from build123d import *

# Parameters (mm, degrees)
SKETCH3_W           = 13
SKETCH3_H           = 120
BOSS_EXTRUDE1_DEPTH = 4
SKETCH11_W          = 33
SKETCH11_H          = 120
BOSS_EXTRUDE4_DEPTH = 4
SKETCH12_R          = 2.5
CUT_EXTRUDE3_DEPTH  = 76.305579191
SKETCH13_W          = 6.102814475
SKETCH13_H          = 45
CUT_EXTRUDE4_DEPTH  = 76.305579191


with BuildPart() as part:
    # Sketch3 → Boss-Extrude1 (new body)
    with BuildSketch(Plane.XY):
        with Locations((20.835766423, 0)):
            Rectangle(SKETCH3_W, SKETCH3_H)
        with BuildLine():
            Line((14.335766423, 0), (14.335766423, 60))
            Line((14.335766423, 60), (-22.664233577, 60))
            ThreePointArc((-22.664233577, 60), (-0.008037132, 46.062450015), (12.335766423, 22.5))
            Line((12.335766423, 22.5), (12.335766423, 0))
            Line((12.335766423, 0), (14.335766423, 0))
        make_face()
        with BuildLine():
            Line((14.335766423, -60), (14.335766423, 0))
            Line((14.335766423, 0), (12.335766423, 0))
            Line((12.335766423, 0), (12.335766423, -22.5))
            ThreePointArc((12.335766423, -22.5), (-0.008037132, -46.062450015), (-22.664233577, -60))
            Line((-22.664233577, -60), (14.335766423, -60))
        make_face()
    extrude(amount=BOSS_EXTRUDE1_DEPTH)


with BuildPart() as body_2:
    # Mirror4: mirrored copy
    add(part.part.mirror(Plane.XY.offset(-12.5)))


with BuildPart() as part_1:
    add(part.part)

    add(body_2.part)  # Boss-Extrude4 merges body 2
    # Sketch11 → Boss-Extrude4 (add)
    with BuildSketch(Plane(origin=(27.335766423, 0, 0), x_dir=(0, 0, -1), z_dir=(1, 0, 0))):
        with Locations((12.5, 0)):
            Rectangle(SKETCH11_W, SKETCH11_H)
    extrude(amount=BOSS_EXTRUDE4_DEPTH)

    # Sketch12 → Cut-Extrude3 (cut, through all)
    with BuildSketch(Plane.XY.offset(4)):
        with Locations((10.835766423, 52.5)):
            Circle(SKETCH12_R)
    cut_extrude3 = extrude(amount=-CUT_EXTRUDE3_DEPTH, mode=Mode.SUBTRACT)

    # Mirror5: Cut-Extrude3 across plane
    add(cut_extrude3.mirror(Plane.ZX), mode=Mode.SUBTRACT)

    # Sketch13 → Cut-Extrude4 (cut, through all)
    with BuildSketch(Plane.XY.offset(4)):
        with Locations((24.835766424, 0)):
            Rectangle(SKETCH13_W, SKETCH13_H)
    extrude(amount=-CUT_EXTRUDE4_DEPTH, mode=Mode.SUBTRACT)


solid = part_1.part
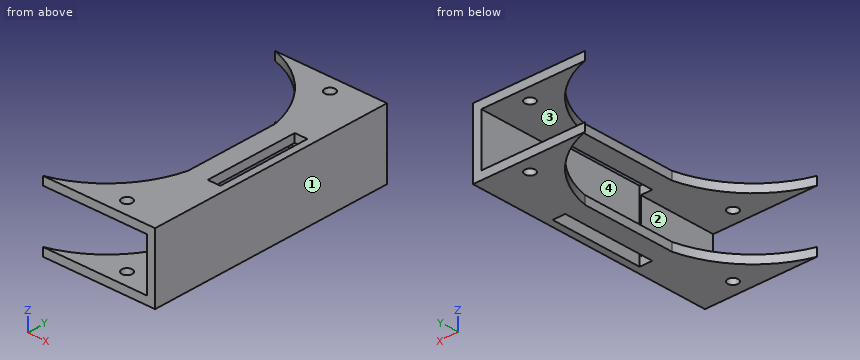
The model under review builds one solid part; all positions refer to its coordinate system, in mm. Face numbers are marked on the shaded views. A direction names the side the tool comes from. Round coordinates to 2 decimals unless told otherwise and drop trailing zeros. Loops run counter-clockwise (first coordinate to the right, second up) from the corner with the lowest first, then second, coordinate; pieces in that order, holes last. Notation, with made-up numbers: (83.5, 50) -> (130.5, 50) arc R28 ccw to (130.5, 74) -> close; hole circle Ø5 at (0, -36.5). An arc over 180 degrees is marked (long way). One line per question, with ' | ' between items. Start each with the question number.
Item 1: Wall thickness on line 1 along Z through (x, y) = (15.5, -26); line 2 along X through (y, z) = (14.5, -27); line 3 along X through (y, z) = (38.5, -16.5): over which ranges is each line inside the solid? List them lowest first. Write a range as [from, to].
Item 2: Add section B-B, the plane x = 23.5. Write out the cut boundary in (y, z), then the cut area to 3 significant figures.
Item 3: Add section A-A, the plane x = 15.5. Write out the cut boundary in (y, z), then the cut area to 3 significant figures.
Item 4: Draft analysis for pull direction Y (two halves, no side actions). For the marked faces 3 and 4, state which applies: +Y half, -Y half, draft (parallel to the pull), parting line (faces both ways), or undercut.
Item 5: Add section D-D, the plane y = -52.5. Write out the cut boundary in (x, z), then the cut area to 3 significant figures.
Item 6: Add section C-C, the plane z = -21.5. Write out the cut boundary in (x, y).
Item 7: For pin 1 (4.5 mm diameter, centred on y = 6, z = 1.5, fed in from -X); pin 2 (12.5 mm diameter, centred on y = -48, z = -13.5, fed in from -X); pin 3 (10 mm diameter, centred on y = -10, z = -14, fed in from -X), all flat-tipped, find the tip position at first contact; note any pin that passes through.
Item 8: Machinability: for the marked faces 1 and 2, which of the approach directions +Z, -Z, +X, -X, +Y, -Y give a long, thin tool a straight path to every point of the face, cutting with its end or side? Answer none if there is none.
Return value:
1) line 1: z = [-29, -25], [0, 4] | line 2: x = [12.34, 21.78], [27.89, 31.34] | line 3: x = [27.34, 31.34]
2) outline: (-60, -29) -> (-22.5, -29) -> (-22.5, -25) -> (-60, -25) -> close; (-60, 0) -> (-22.5, 0) -> (-22.5, 4) -> (-60, 4) -> close; (22.5, -29) -> (60, -29) -> (60, -25) -> (22.5, -25) -> close; (22.5, 0) -> (60, 0) -> (60, 4) -> (22.5, 4) -> close | area: 600 mm2
3) outline: (-60, -29) -> (60, -29) -> (60, -25) -> (-60, -25) -> close; (-60, 0) -> (60, 0) -> (60, 4) -> (-60, 4) -> close | area: 960 mm2
4) face 3: draft | face 4: undercut
5) outline: (-7.31, -29) -> (8.34, -29) -> (8.34, -25) -> (-7.31, -25) -> close; (-7.31, 0) -> (8.34, 0) -> (8.34, 4) -> (-7.31, 4) -> close; (13.34, -29) -> (31.34, -29) -> (31.34, 4) -> (13.34, 4) -> (13.34, 0) -> (27.34, 0) -> (27.34, -25) -> (13.34, -25) -> close | area: 369 mm2
6) outline: (27.34, -60) -> (31.34, -60) -> (31.34, 60) -> (27.34, 60) -> (27.34, 22.5) -> (27.89, 22.5) -> (27.89, -22.5) -> (27.34, -22.5) -> close
7) pin 1: stops at x = 12.34 | pin 2: stops at x = 27.34 | pin 3: stops at x = 27.89
8) face 1: +Z, -Z, +X, +Y, -Y | face 2: -X, +Y, -Y
